```python
from build123d import *

# Parameters (mm, degrees)
SKETCH1_R           = 16
SKETCH1_R_2         = 1.6
BOSS_EXTRUDE1_DEPTH = 3.175
SKETCH2_R           = 6.05
BOSS_EXTRUDE2_DEPTH = 3.175


with BuildPart() as part:
    # Sketch1 → Boss-Extrude1 (new body)
    with BuildSketch(Plane(origin=(0, 0, 0), x_dir=(0, 0, -1), z_dir=(1, 0, 0))):
        Circle(SKETCH1_R)
        with Locations((0, 11.313708499)):
            Circle(SKETCH1_R_2, mode=Mode.SUBTRACT)
        with Locations((11.313708499, 0)):
            Circle(SKETCH1_R_2, mode=Mode.SUBTRACT)
        with Locations((0, -11.313708499)):
            Circle(SKETCH1_R_2, mode=Mode.SUBTRACT)
        with Locations((-11.313708499, 0)):
            Circle(SKETCH1_R_2, mode=Mode.SUBTRACT)
    extrude(amount=BOSS_EXTRUDE1_DEPTH)

    # Sketch2 → Boss-Extrude2 (add)
    with BuildSketch(Plane(origin=(3.175, 0, 0), x_dir=(0, 0, -1), z_dir=(1, 0, 0))):
        Circle(SKETCH2_R)
    extrude(amount=BOSS_EXTRUDE2_DEPTH)


solid = part.part
```
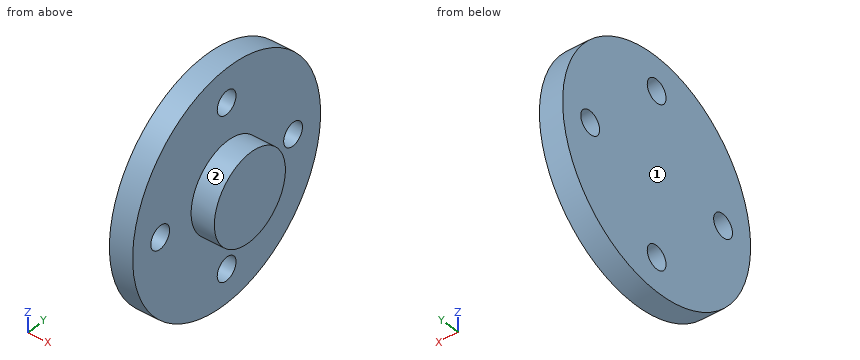
Verification items for the finished model (mm, model axes). Face numbers are marked on the shaded views. A direction names the side the tool comes from. Round coordinates to 2 decimals unless told otherwise and drop trailing zeros. Loops run counter-clockwise (first coordinate to the right, second up) from the corner with the lowest first, then second, coordinate; pieces in that order, holes last. Notation, with made-up numbers: (6.5, 57.25) -> (43.5, 57.25) arc R23 cw to (43.5, 73.25) -> close; hole circle Ø5 at (-25.75, 35.25). An arc over 180 degrees is marked (long way). Answer as a JSON object with one key per item and string values.
Q1. Section check D-D (y = 12). Record the boundary of the cut face in (x, z) (3 decimals).
Data:
{"outline": "(0, -10.583) -> (3.175, -10.583) -> (3.175, -1.445) -> (0, -1.445) -> close; (0, 1.445) -> (3.175, 1.445) -> (3.175, 10.583) -> (0, 10.583) -> close"}
Q2. Section check A-A (z = 0). Record the boundary of the cut face in (x, y) (3 decimals).
Data:
{"outline": "(0, -16) -> (3.175, -16) -> (3.175, -12.914) -> (0, -12.914) -> close; (0, -9.714) -> (3.175, -9.714) -> (3.175, -6.05) -> (6.35, -6.05) -> (6.35, 6.05) -> (3.175, 6.05) -> (3.175, 9.714) -> (0, 9.714) -> close; (0, 12.914) -> (3.175, 12.914) -> (3.175, 16) -> (0, 16) -> close"}
Q3. Access from +Z, -Z, +X, -X, +Y, -Y to the whole of each face (thin tool, end or side, straight path). Record for the marked faces 1 and 2.
Data:
{"face 1": "+Z, -Z, -X, +Y, -Y", "face 2": "+X"}
Q4. Go/stop test with flat-tipped pins: P1, Ø5, axis at y = -12, z = 7.5, coming from the -X side; P2, Ø3.5, axis at y = 0, z = -11.31, coming from the +X side (3 decimals). Record where each tip stops, or that it passes through.
Data:
{"P1": "stops at x = 0", "P2": "stops at x = 3.175"}
Q5. Section check C-C (z = -11.5). Record the boundary of the cut face in (x, y) (3 decimals), then the cut area to 3 significant figures.
Data:
{"outline": "(0, -11.124) -> (3.175, -11.124) -> (3.175, -1.589) -> (0, -1.589) -> close; (0, 1.589) -> (3.175, 1.589) -> (3.175, 11.124) -> (0, 11.124) -> close", "area": "60.5 mm2"}
Q6. Scan lines: line 1 (Y direction, x = 1.25, z = 0); line 2 (X direction, y = 2, z = -10) (3 decimals); line 3 (Y direction, x = 2.5, z = 12). Record each from-to range of solid material in increasing order. Write a range as from..to.
Data:
{"line 1": "y = -16..-12.91, -9.71..9.71, 12.91..16", "line 2": "x = 0..3.175", "line 3": "y = -10.58..-1.45, 1.45..10.58"}
